```python
from build123d import *

# Parameters (mm, degrees)
ESQUISSE1_W                         = 45
ESQUISSE1_H                         = 22
BOSS_EXTRU_1_DEPTH                  = 4
ESQUISSE2_R                         = 6.4
ENL_V_MAT_EXTRU_1_DEPTH             = 4
FILETAGE1_PITCH                     = 1.4
ESQUISSE3_W                         = 4
ESQUISSE3_H                         = 22
BOSS_EXTRU_2_DEPTH                  = 10
ESQUISSE4_W                         = 3
ESQUISSE4_H                         = 22
BOSS_EXTRU_3_DEPTH                  = 37
ENL_V_MAT_EXTRU_2_REACH             = 49.592
ESQUISSE5_R                         = 3.25
ENL_V_MAT_EXTRU_2_DIRECTION_2_REACH = 49.592
ESQUISSE6_W                         = 45
ESQUISSE6_H                         = 4
BOSS_EXTRU_4_DEPTH                  = 25
ESQUISSE7_R                         = 8
ENL_V_MAT_EXTRU_4_DEPTH             = 25
ESQUISSE8_W                         = 14
ESQUISSE8_H                         = 4
BOSS_EXTRU_5_DEPTH                  = 4.5


with BuildPart() as part:
    # Esquisse1 → Boss.-Extru.1 (new body)
    with BuildSketch(Plane.XY):
        with Locations((22.5, -11)):
            Rectangle(ESQUISSE1_W, ESQUISSE1_H)
    extrude(amount=BOSS_EXTRU_1_DEPTH)

    # Esquisse2 → Enlèv. mat.-Extru.1 (cut)
    with BuildSketch(Plane(origin=(0, 0, 0), x_dir=(-1, 0, 0), z_dir=(0, 0, -1))):
        with Locations((-15, -11)):
            Circle(ESQUISSE2_R)
    extrude(amount=-ENL_V_MAT_EXTRU_1_DEPTH, mode=Mode.SUBTRACT)

    # Filetage1: the profile of Profil de filetage1 profile screwed along a right-hand helix of 4 turns, 8 arcs to a turn; built about Z, then put on its axis
    filetage1_z = Axis((0, 0, 0), (0, 0, 1))
    filetage1_corners = [(6.3997, 0, -0.000173205), (7.211898812, 0, 0.468749998), (7.211898812, 0, 0.656249998), (6.3997, 0, 1.125173201)]
    with BuildLine(mode=Mode.PRIVATE) as filetage1_profile:
        Line(filetage1_corners[0], filetage1_corners[1])
        Line(filetage1_corners[1], filetage1_corners[2])
        Line(filetage1_corners[2], filetage1_corners[3])
        Line(filetage1_corners[3], filetage1_corners[0])
    filetage1_cap = Face(filetage1_profile.wire())
    filetage1_turn_angles = [0, 22.5, 45, 67.5, 90, 112.5, 135, 157.5, 180, 202.5, 225, 247.5, 270, 292.5, 315, 337.5, 360]
    filetage1_turn_weights = [1, 0.9238795325112867, 1, 0.9238795325112867, 1, 0.9238795325112867, 1, 0.9238795325112867, 1, 0.9238795325112867, 1, 0.9238795325112867, 1, 0.9238795325112867, 1, 0.9238795325112867, 1]
    filetage1_turn_rails = [Edge.make_bspline([Vector(p[0], p[1], 0).rotate(filetage1_z, filetage1_turn_angles[k]) / filetage1_turn_weights[k] + Vector(0, 0, p[2] + FILETAGE1_PITCH * filetage1_turn_angles[k] / 360) for k in range(17)], [0, 0, 0, 1, 1, 2, 2, 3, 3, 4, 4, 5, 5, 6, 6, 7, 7, 8, 8, 8], 2, filetage1_turn_weights) for p in filetage1_corners]
    filetage1_turn_sides = [Face.make_surface_from_curves(filetage1_turn_rails[p[0]], filetage1_turn_rails[p[1]]) for p in [(0, 1), (1, 2), (2, 3), (3, 0)]]
    filetage1 = Plane(origin=(15, -11, -1), x_dir=(1, 0, 0), z_dir=(0, 0, 1)) * Solid(Shell([*[p.moved(Location((0, 0, FILETAGE1_PITCH * i))) for i in range(4) for p in filetage1_turn_sides], filetage1_cap, filetage1_cap.rotate(filetage1_z, 1440).moved(Location((0, 0, FILETAGE1_PITCH * 1440 / 360)))]))
    add(filetage1, mode=Mode.SUBTRACT)

    # Esquisse3 → Boss.-Extru.2 (add)
    with BuildSketch(Plane(origin=(0, 0, 0), x_dir=(-1, 0, 0), z_dir=(0, 0, -1))):
        with Locations((-43, -11)):
            Rectangle(ESQUISSE3_W, ESQUISSE3_H)
        with Locations((-2, -11)):
            Rectangle(ESQUISSE3_W, ESQUISSE3_H)
    extrude(amount=BOSS_EXTRU_2_DEPTH)

    # Esquisse4 → Boss.-Extru.3 (add)
    with BuildSketch(Plane(origin=(4, 0, 0), x_dir=(0, 0, -1), z_dir=(1, 0, 0))):
        with Locations((8.5, -11)):
            Rectangle(ESQUISSE4_W, ESQUISSE4_H)
    extrude(amount=BOSS_EXTRU_3_DEPTH)

    # Enlèv. mat.-Extru.2: up to this face of the body (flat: up to its plane)
    enl_v_mat_extru_2_end = Plane(part.part.faces().sort_by_distance((0, -11, -3))[0])
    # Esquisse5 → Enlèv. mat.-Extru.2 (cut, up to the picked face)
    with BuildSketch(Plane(origin=(4, 0, 0), x_dir=(0, 0, -1), z_dir=(1, 0, 0)), mode=Mode.PRIVATE) as enl_v_mat_extru_2_sk1:
        with Locations(Location((3.75, -11, 0), (0, 0, 180))):
            Circle(ESQUISSE5_R)
    enl_v_mat_extru_2_tool1 = split(extrude(enl_v_mat_extru_2_sk1.sketch, amount=-ENL_V_MAT_EXTRU_2_REACH, mode=Mode.PRIVATE), bisect_by=enl_v_mat_extru_2_end, keep=Keep.BOTH, mode=Mode.PRIVATE)
    add(enl_v_mat_extru_2_tool1.solids().sort_by(Axis((4, -11, -3.75), (-1, 0, 0)))[0], mode=Mode.SUBTRACT)

    # Enlèv. mat.-Extru.2 direction 2: up to this face of the body (flat: up to its plane)
    enl_v_mat_extru_2_direction_2_end = Plane(part.part.faces().sort_by_distance((45, -11, -3))[0])
    # Esquisse5 → Enlèv. mat.-Extru.2 direction 2 (cut, up to the picked face)
    with BuildSketch(Plane(origin=(4, 0, 0), x_dir=(0, 0, -1), z_dir=(1, 0, 0)), mode=Mode.PRIVATE) as enl_v_mat_extru_2_direction_2_sk1:
        with Locations(Location((3.75, -11, 0), (0, 0, 180))):
            Circle(ESQUISSE5_R)
    enl_v_mat_extru_2_direction_2_tool1 = split(extrude(enl_v_mat_extru_2_direction_2_sk1.sketch, amount=ENL_V_MAT_EXTRU_2_DIRECTION_2_REACH, mode=Mode.PRIVATE), bisect_by=enl_v_mat_extru_2_direction_2_end, keep=Keep.BOTH, mode=Mode.PRIVATE)
    add(enl_v_mat_extru_2_direction_2_tool1.solids().sort_by(Axis((4, -11, -3.75), (1, 0, 0)))[0], mode=Mode.SUBTRACT)

    # Esquisse6 → Boss.-Extru.4 (add)
    with BuildSketch(Plane.XY.offset(4)):
        with Locations((22.5, -2)):
            Rectangle(ESQUISSE6_W, ESQUISSE6_H)
        with Locations((22.5, -20)):
            Rectangle(ESQUISSE6_W, ESQUISSE6_H)
    extrude(amount=BOSS_EXTRU_4_DEPTH)

    # Esquisse7 → Enlèv. mat.-Extru.4 (cut)
    with BuildSketch(Plane.XY.offset(4)):
        with Locations((15, -11)):
            Circle(ESQUISSE7_R)
    extrude(amount=ENL_V_MAT_EXTRU_4_DEPTH, mode=Mode.SUBTRACT)

    # Esquisse8 → Boss.-Extru.5 (add)
    with BuildSketch(Plane(origin=(45, 0, 0), x_dir=(0, 0, -1), z_dir=(1, 0, 0))):
        with Locations((3, -20)):
            Rectangle(ESQUISSE8_W, ESQUISSE8_H)
        with Locations((3, -2)):
            Rectangle(ESQUISSE8_W, ESQUISSE8_H)
    extrude(amount=BOSS_EXTRU_5_DEPTH)


solid = part.part
```
Work out the finished part from the listing and answer in its coordinate system (mm). A direction names the side the tool comes from. Give positions to 0.01 mm unless a question says otherwise; leave off trailing zeros. Loops run counter-clockwise (first coordinate to the right, second up) from the corner with the lowest first, then second, coordinate; pieces in that order, holes last. Notation, with made-up numbers: M -8.75,24.5 L 32.25,24.5 A26 ccw 32.25,50.5 Z; hole C 0,63.25 d5. An arc over 180 degrees is marked long. One line per item, written item: value. Start each with the question number.
1. Each of these flat-tipped pins is pushed along its axis until it touches: P1, Ø11.5, axis at x = 15, y = -11, coming from the +Z side; P2, Ø4, axis at y = -4, z = 16, coming from the +X side; P3, Ø1, axis at x = 6.5, y = -5.5, coming from the +Z side. Where does it stop, or does it pass through?
2. Find section C-C (y = -1.5). Give the vertices of the cut face in (x, z).
3. Determine the mould class of faces 1 (the face through (45, -20, 16)), 2 (the face through (22, -11, 0)), 3 (the face through (24, -11, -10)) for opening direction X: released by +X, released by -X, zero draft, split by the parting line, or undercut.
4. Find section A-A (z = -3.75). Give the vertices of the cut face in (x, y).
5. Which of the six approach directions +Z, -Z, +X, -X, +Y, -Y give full straight-line access (tool end or side, diameter ignored) to faces 4 (the face through (15, -19, 16)), 5 (the face through (47, -4, -3)), 6 (the face through (5, -18, 16))?
6. Find the intervals of material crossed by probe 1 along Z at (x, y) = (31.5, -5.75); probe 2 along X at (y, z) = (-11, 0.9); probe 3 along Y at (x, z) = (0.85, -3.75), in increasing order.
7. Find section D-D (z = 11). Give the vertices of the cut face in (x, y), and give its area (3 significant figures).
8. Find section B-B (x = 34.5). Give the vertices of the cut face in (y, z).
Reported:
1. P1: stops at z = -7
1. P2: stops at x = 45
1. P3: stops at z = 4
2. outline: M 0,-10 L 49.5,-10 L 49.5,4 L 45,4 L 45,29 L 0,29 Z; hole M 4,-7 L 41,-7 L 41,0 L 4,0 Z
3. face 1: released by +X
3. face 2: undercut
3. face 3: zero draft
4. outline: M 0,-22 L 4,-22 L 4,-14.25 L 0,-14.25 Z; M 0,-7.75 L 4,-7.75 L 4,0 L 0,0 Z; M 41,-22 L 49.5,-22 L 49.5,-18 L 45,-18 L 45,-14.25 L 41,-14.25 Z; M 41,-7.75 L 45,-7.75 L 45,-4 L 49.5,-4 L 49.5,0 L 41,0 Z
5. face 4: +Z
5. face 5: +Z, -Z, +X
5. face 6: +Z, +X, -X
6. probe 1: z = -10 to -7, 0 to 4
6. probe 2: x = 0 to 8.6, 22.21 to 45
6. probe 3: y = -22 to -14.25, -7.75 to 0
7. outline: M 0,-22 L 45,-22 L 45,-18 L 18.87,-18 A8 cw 11.13,-18 L 0,-18 Z; M 0,-4 L 11.13,-4 A8 cw 18.87,-4 L 45,-4 L 45,0 L 0,0 Z
7. area: 350 mm²
8. outline: M -22,-10 L 0,-10 L 0,-7 L -22,-7 Z; M -22,0 L 0,0 L 0,29 L -4,29 L -4,4 L -18,4 L -18,29 L -22,29 Z
